```python
from build123d import *

# Parameters (mm, degrees)
F1_DEPTH = 10
F2_W     = 30
F2_H     = 100
F3_DEPTH = 100
F4_SIZE  = 99.99999


# Not quite as in the source:
# - a fillet or chamfer is up to 0.001 mm smaller than in the source, because OpenCascade refuses the exact size


with BuildPart() as f1:
    # F0 (on Front) → F1 (new body)
    with BuildSketch(Plane.XZ):
        Polygon((0, -100), (0, 0), (-100, 0), (-15, -100), align=None)
        Polygon((100, 0), (0, 0), (0, -100), (15, -100), align=None)
    extrude(amount=F1_DEPTH)

    # F2 (on face) → F3 (join)
    with BuildSketch(Plane.XZ.offset(10)):
        with Locations((0, -50)):
            Rectangle(F2_W, F2_H)
    extrude(amount=F3_DEPTH)

    # F4 (size 100 in the source; OpenCascade refuses exactly that, so slightly less here)
    f4_edges = [f1.edges().sort_by_distance(p)[0] for p in [
        (0, -110, -100),
    ]]
    chamfer(f4_edges, length=F4_SIZE)


solid = f1.part
```
Design review of the part built by this model. Coordinates are the model's own, in mm. A direction names the side the tool comes from. Coordinates: 2 decimals unless noted, no trailing zeros. Loops run counter-clockwise (first coordinate to the right, second up) from the corner with the lowest first, then second, coordinate; pieces in that order, holes last.
Q1. We need section A-A on z = -87.5. State the section outline as (x, y) points (3 decimals), and give its area (4 significant figures).
Reported:
outline: (-25.625, -10) - (-15, -10) - (-15, -22.5) - (15, -22.5) - (15, -10) - (25.625, -10) - (25.625, 0) - (-25.625, 0) - close
area: 887.5 mm2
Q2. To check wall thickness, follow line 1 (X direction, y = -51.5, z = -31); line 2 (Y direction, x = -28, z = -74); line 3 (Y direction, x = -10, z = -71.5). State the ranges of each line that lie inside material, in increasing order.
Reported:
line 1: x = -15 to 15
line 2: y = -10 to 0
line 3: y = -38.5 to 0
Q3. Tool access review of faces 1 (the face through (0, -5, -100)), 2 (the face through (47, -10, -38)), 3 (the face through (-15, -48, -40)): name each direction out of +Z, -Z, +X, -X, +Y, -Y from which nothing blocks a thin tool from reaching the whole face with its end or side.
Reported:
face 1: -Z, +X, -X, +Y, -Y
face 2: +Z, -Z, +X, -Y
face 3: +Z, -Z, -X, -Y
Q4. We need section C-C on x = -17. State the section outline as (y, z) points.
Reported:
outline: (-10, -97.65) - (0, -97.65) - (0, 0) - (-10, 0) - close
Q5. For pin 1 (1.5 mm diameter, centred on y = -95, z = -11.5, fed in from +X); pin 2 (6 mm diameter, centred on x = 15.5, z = -33.5, fed in from +Y); pin 3 (8 mm diameter, centred on y = -48.5, z = -10.5, fed in from -X); pin 4 (2 mm diameter, centred on x = -4.5, z = -74.5, fed in from -Y), all flat-tipped, find the tip position at first contact; note any pin that passes through.
Reported:
pin 1: stops at x = 15
pin 2: stops at y = 0
pin 3: stops at x = -15
pin 4: stops at y = -36.5
Q6. We need section D-D on z = -56.5. State the section outline as (x, y) points (3 decimals), and give its area (3 significant figures).
Reported:
outline: (-51.975, -10) - (-15, -10) - (-15, -53.5) - (15, -53.5) - (15, -10) - (51.975, -10) - (51.975, 0) - (-51.975, 0) - close
area: 2,340 mm2
Q7. We need section B-B on y = -91. State the section outline as (x, z) points.
Reported:
outline: (-15, -19) - (15, -19) - (15, 0) - (-15, 0) - close
